Part model, mm, in its own coordinate system. Coordinates: 2 decimals unless noted, no trailing zeros. Loops run counter-clockwise (first coordinate to the right, second up) from the corner with the lowest first, then second, coordinate; pieces in that order, holes last. Notation, with made-up numbers: (89, 11) - (130, 11) arc R9 ccw to (130, 22) - close; hole circle Ø8 at (9, 76.5). An arc over 180 degrees is marked (long way). Use a Markdown table: item, result. Add a question column.
1) Probe probe 1 along Z at (x, y) = (1.7, 4.5); probe 2 along Y at (x, z) = (2.85, -4.5); probe 3 along Z at (x, y) = (1.3, 3.75). List the from-to ranges inside material, lowest first. Write a range as [from, to].
2) Band-saw the part on C-C (z = -4.5). Give the cut face in (x, y), plus the area to 3 significant figures.
3) Band-saw the part on D-D (z = -44.5). Give the cut face in (x, y), plus the area to 3 significant figures.
4) Band-saw the part on A-A (y = 4.5). Give the cut face in (x, z), plus the area to 3 significant figures.
5) Pull direction Z, two halves, no side cores. Call faces 1 (the face through (0.127, 0.387, -0.373)), 2 (the face through (1.972, 5.266, -47.347)), 3 (the face through (0.127, 0.373, -49.613)): +Z half, -Z half, draft (parallel to the pull), parting line (faces both ways), or undercut.
6) Band-saw the part on B-B (x = 2.5). Give the cut face in (y, z), plus the area to 3 significant figures.
Autodesk Inventor part; units mm, degrees
ref_plane "YZ Plane" through (0, 0, 0) normal (1, 0, 0) x (0, 1, 0)
ref_plane "XZ Plane" through (0, 0, 0) normal (0, 1, 0) x (-1, 0, 0)
ref_plane "XY Plane" through (0, 0, 0) normal (0, 0, 1) x (1, 0, 0)
sketch "Sketch1" plane through (0, 0, 0) normal (0, 0, 1) x (1, 0, 0)
  line L0 (0, 0) -> (4, 0)
  line L1 (4, 0) -> (4, 9)
  line L2 (4, 9) -> (0, 9)
  line L3 (0, 9) -> (0, 0)
  dimension "d3" = 4
  dimension "d4" = 9
extrude "Extrusion1" add sketch "Sketch1" against normal blind 50
sketch "Sketch2" plane through (4, 0, 0) normal (1, 0, 0) x (0, 0, -1)
  circle A0 centre (4.5, 4.5) radius 2
  circle A1 centre (45.5, 4.5) radius 2
  line L0 (0, 0) -> (50, 0)
  line L1 (0, 0) -> (0, 9)
  line L2 (50, 9) -> (50, 0)
  line L3 (0, 9) -> (50, 9)
  dimension "d7" = 4
  dimension "d8" = 4
  dimension "d9" = 4.5
  dimension "d10" = 4.5
  dimension "d11" = 41
  dimension "d12" = 4.5
  dimension "d13" = 4.5
hole "Hole1" at (4, 4.5, -4.5) at (4, 4.5, -45.5) direction (-1, 0, 0) diameter 4 depth 4 tip angle 118
fillet "Fillet1" radius 1 4 edges at (2, 9, 0) (2, 0, 0) (2, 9, -50) (2, 0, -50)
chamfer "Chamfer1" distance 0.25 angle 45 16 edges at (0, 9, -25) (0, 8.7071, -49.7071) (0, 4.5, -50) (0, 0.2929, -49.7071) (0, 0, -25) (0, 0.2929, -0.2929) (0, 4.5, 0) (0, 8.7071, -0.2929) (4, 0, -25) (4, 0.2929, -49.7071) (4, 4.5, -50) (4, 8.7071, -49.7071) (4, 9, -25) (4, 8.7071, -0.2929) (4, 4.5, 0) (4, 0.2929, -0.2929)
properties part number "HUDSON 1-03 AXLE BOX KEEPER"
Answer block:
| question | item | result |
|---|---|---|
| 1 | probe 1 | [-50, -47.5], [-43.5, -6.5], [-2.5, 0] |
| 1 | probe 2 | [0, 2.5], [6.5, 9] |
| 1 | probe 3 | [-50, -47.35], [-43.65, -6.35], [-2.65, 0] |
| 2 | outline | (0, 0.25) - (0.25, 0) - (3.75, 0) - (4, 0.25) - (4, 2.5) - (0, 2.5) - close; (0, 6.5) - (4, 6.5) - (4, 8.75) - (3.75, 9) - (0.25, 9) - (0, 8.75) - close |
| 2 | area | 19.9 mm2 |
| 3 | outline | (0, 0.25) - (0.25, 0) - (3.75, 0) - (4, 0.25) - (4, 2.77) - (0, 2.77) - close; (0, 6.23) - (4, 6.23) - (4, 8.75) - (3.75, 9) - (0.25, 9) - (0, 8.75) - close |
| 3 | area | 22.0 mm2 |
| 4 | outline | (0, -49.75) - (0.25, -50) - (3.75, -50) - (4, -49.75) - (4, -47.5) - (0, -47.5) - close; (0, -43.5) - (4, -43.5) - (4, -6.5) - (0, -6.5) - close; (0, -2.5) - (4, -2.5) - (4, -0.25) - (3.75, 0) - (0.25, 0) - (0, -0.25) - close |
| 4 | area | 168 mm2 |
| 5 | face 1 | +Z half |
| 5 | face 2 | undercut |
| 5 | face 3 | -Z half |
| 6 | outline | (0, -49) arc R1 ccw to (1, -50) - (8, -50) arc R1 ccw to (9, -49) - (9, -1) arc R1 ccw to (8, 0) - (1, 0) arc R1 ccw to (0, -1) - close; hole circle Ø4 at (4.5, -45.5); hole circle Ø4 at (4.5, -4.5) |
| 6 | area | 424 mm2 |
